Check sheet for the modelled part. Datum: model origin and axes. Units: mm. A direction names the side the tool comes from. Give positions to 0.01 mm unless a question says otherwise; leave off trailing zeros. Loops run counter-clockwise (first coordinate to the right, second up) from the corner with the lowest first, then second, coordinate; pieces in that order, holes last. Notation, with made-up numbers: M -40,16 L -32,16 A28 cw -32,50 Z; hole C 74,74.5 d8. An arc over 180 degrees is marked long. Put each result on its own line as item: value. Start each with the question number.
Autodesk Inventor part; units mm, degrees
ref_plane "YZ Plane" through (0, 0, 0) normal (1, 0, 0) x (0, 1, 0)
ref_plane "XZ Plane" through (0, 0, 0) normal (0, 1, 0) x (-1, 0, 0)
ref_plane "XY Plane" through (0, 0, 0) normal (0, 0, 1) x (1, 0, 0)
sketch "スケッチ1" plane through (0, 0, 0) normal (0, 0, 1) x (1, 0, 0)
  circle A0 centre (0, 0) radius 5.95
  dimension "d0" = 11.9
extrude "押し出し1" add sketch "スケッチ1" along normal blind 188
thread "ねじ1"
sketch "スケッチ3" plane through (0, 0, 188) normal (0, 0, 1) x (1, 0, 0)
  circle A0 centre (0, 0) radius 11.3
  dimension "d5" = 22.6
extrude "押し出し2" add sketch "スケッチ3" along normal blind 4.5
sketch "スケッチ4" plane through (0, 0, 192.5) normal (0, 0, 1) x (1, 0, 0)
  circle A0 centre (0, 0) radius 5.95 construction
  line L0 (5.95, -3.4352) -> (0, -6.8705)
  line L1 (0, -6.8705) -> (-5.95, -3.4352)
  line L2 (-5.95, -3.4352) -> (-5.95, 3.4352)
  line L3 (-5.95, 3.4352) -> (0, 6.8705)
  line L4 (0, 6.8705) -> (5.95, 3.4352)
  line L5 (5.95, 3.4352) -> (5.95, -3.4352)
  point P0 (5.95, 0)
extrude "押し出し3" add sketch "スケッチ4" along normal blind 6.3
properties part number "前輪シャフト"
Q1. Section check B-B, the plane z = 96. Record the cut outline in (x, y).
Q2. Access from +Z, -Z, +X, -X, +Y, -Y to the whole of each face (thin tool, end or side, straight path). Record for faces 1 (the face through (5, -5, 188)), 2 (the face through (5, -5, 192.5)), 3 (the face through (3.017, -5.129, 195.606)).
Q3. Section check C-C, the plane x = 4. Record the cut outline in (y, z), then the cut area to 3 significant figures.
Q4. Section check A-A, the plane y = 0. Record the cut outline in (x, z), then the cut area to 3 significant figures.
Q5. Depth check by flat-ended pin: P1, Ø5, axis at y = 6.5, z = 99.5, coming from the -X side; P2, Ø12, axis at y = -8.5, z = 102.5, coming from the -X side; P3, Ø10, axis at y = -0.5, z = 83, coming from the +X side. Enter the tip coordinate at first touch or a pass-through.
Q6. Thickness scan on line 1 along Z through (x, y) = (6.5, -4); line 2 along X through (y, z) = (-0.5, 95); line 3 along X through (y, z) = (-2.75, 68). Record the ranges inside material, lowest first. Write a range as [from, to].
Q7. Section check D-D, the plane y = -9.5. Record the cut outline in (x, z).
Found:
1. outline: C 0,0 d11.9
2. face 1: -Z
2. face 2: +Z
2. face 3: +Z, +X, -Y
3. outline: M -10.57,188 L -4.4,188 L -4.4,0 L 4.4,0 L 4.4,188 L 10.57,188 L 10.57,192.5 L 4.56,192.5 L 4.56,198.8 L -4.56,198.8 L -4.56,192.5 L -10.57,192.5 Z
3. area: 1,810 mm^2
4. outline: M -11.3,188 L -5.95,188 L -5.95,0 L 5.95,0 L 5.95,188 L 11.3,188 L 11.3,192.5 L 5.95,192.5 L 5.95,198.8 L -5.95,198.8 L -5.95,192.5 L -11.3,192.5 Z
4. area: 2,410 mm^2
5. P1: stops at x = -4.4
5. P2: stops at x = -5.4
5. P3: stops at x = 5.95
6. line 1: z = [188, 192.5]
6. line 2: x = [-5.93, 5.93]
6. line 3: x = [-5.28, 5.28]
7. outline: M -6.12,188 L 6.12,188 L 6.12,192.5 L -6.12,192.5 Z
